Autodesk Inventor part; units mm, degrees
ref_plane "YZ Plane" through (0, 0, 0) normal (1, 0, 0) x (0, 1, 0)
ref_plane "XZ Plane" through (0, 0, 0) normal (0, 1, 0) x (-1, 0, 0)
ref_plane "XY Plane" through (0, 0, 0) normal (0, 0, 1) x (1, 0, 0)
sketch "Sketch1" plane through (0, 0, 0) normal (0, 1, 0) x (-1, 0, 0)
  line L0 (0, 0) -> (-32, 0)
  line L1 (-32, 0) -> (-32, -24)
  line L2 (-32, -24) -> (0, -24)
  line L3 (0, -24) -> (0, 0)
  circle A0 centre (-8.5, -19) radius 2
  circle A1 centre (-23.5, -19) radius 2
  circle A2 centre (-23.5, -5) radius 2
  circle A3 centre (-8.5, -5) radius 2
  line L4 (-16, -24) -> (-16, 0) construction
  line L5 (0, -12) -> (-32, -12) construction
  dimension "d0" = 32
  dimension "d1" = 24
  dimension "x" = 4
  dimension "d3" = 4
  dimension "d4" = 4
  dimension "d5" = 4
  dimension "d6" = 15
  dimension "d7" = 7.5
  dimension "d8" = 14
  dimension "d9" = 7
extrude "Extrusion1" add sketch "Sketch1" along normal blind 10
sketch "Sketch2" plane through (0, 10, 0) normal (0, 1, 0) x (1, 0, 0)
  circle A0 centre (23.5, 5) radius 2
  circle A1 centre (8.5, 19) radius 2
  circle A2 centre (23.5, 19) radius 2
  circle A3 centre (8.5, 5) radius 2
  circle A4 centre (8.5, 19) radius 3
  circle A5 centre (23.5, 19) radius 3
  circle A6 centre (8.5, 5) radius 3
  circle A7 centre (23.5, 5) radius 3
  point P0 (0, 0)
  dimension "d12" = 6
  dimension "d13" = 6
  dimension "d14" = 6
  dimension "d15" = 6
extrude "Extrusion2" cut sketch "Sketch2" against normal blind 2.5 contours A3 | A4 | A5 | A6 | A7
equation "\"d3\" = x"
equation "\"d4\" = x"
equation "\"d5\" = x"
properties part number "WristMotorTensioner"
Could you check a few things on this model? Use its own coordinates, in mm. A direction names the side the tool comes from. Round coordinates to 2 decimals unless told otherwise and drop trailing zeros. Write each loop counter-clockwise with the first axis right and the second up, starting at its lowest first coordinate (ties: lowest second). Pieces come first, ordered by that corner, then holes.
(1) Suppose I cut it at B-B on x = 23.5. Write out the boundary of the cut face in (y, z).
Findings below:
outline: (0, -24) - (10, -24) - (10, -22) - (7.5, -22) - (7.5, -21) - (0, -21) - close; (0, -17) - (7.5, -17) - (7.5, -16) - (10, -16) - (10, -8) - (7.5, -8) - (7.5, -7) - (0, -7) - close; (0, -3) - (7.5, -3) - (7.5, -2) - (10, -2) - (10, 0) - (0, 0) - close
(2) If I drill on probe 1 along Z at (x, y) = (8.5, 4); probe 2 along X at (y, z) = (9, -5); probe 3 along Z at (x, y) = (8.5, 8.3), over which ranges is the centre line in solid material (lowest first)?
Findings below:
probe 1: z = -24 to -21, -17 to -7, -3 to 0
probe 2: x = 0 to 5.5, 11.5 to 20.5, 26.5 to 32
probe 3: z = -24 to -22, -16 to -8, -2 to 0
(3) For pin 1 (5 mm diameter, centred on x = 23.5, z = -5, fed in from -Y); pin 2 (5 mm diameter, centred on x = 8.5, z = -5, fed in from +Y), each with a flat end and sliding along its axis, tell me the tip position at first contact or that it passes through.
Findings below:
pin 1: stops at y = 0
pin 2: stops at y = 7.5
(4) Thinking about a two-plate mould opening in Z: for faces 3 (the face through (16, 5, -24)), 4 (the face through (21, 7.5, -19)), 5 (the face through (16, 10, -12)), which applies, +Z half, -Z half, draft (parallel to the pull), parting line (faces both ways), or undercut?
Findings below:
face 3: -Z half
face 4: undercut
face 5: draft
(5) Which directions (+Z, -Z, +X, -X, +Y, -Y) give clear straight access to the entire face, cutting with the end or side of a thin tool? Please do faces 1 (the face through (0, 5, -12)), 2 (the face through (21.1, 8.8, -17.2)).
Findings below:
face 1: +Z, -Z, -X, +Y, -Y
face 2: +Y
(6) Suppose I cut it at D-D on y = 8. Write out the boundary of the cut face in (x, z).
Findings below:
outline: (0, -24) - (32, -24) - (32, 0) - (0, 0) - close; hole circle Ø6 at (8.5, -19); hole circle Ø6 at (8.5, -5); hole circle Ø6 at (23.5, -19); hole circle Ø6 at (23.5, -5)
(7) Suppose I cut it at C-C on y = 3.25. Write out the boundary of the cut face in (x, z), and give its area (3 significant figures).
Findings below:
outline: (0, -24) - (32, -24) - (32, 0) - (0, 0) - close; hole circle Ø4 at (8.5, -19); hole circle Ø4 at (8.5, -5); hole circle Ø4 at (23.5, -19); hole circle Ø4 at (23.5, -5)
area: 718 mm2
(8) Suppose I cut it at A-A on z = -5. Write out the boundary of the cut face in (x, y).
Findings below:
outline: (0, 0) - (6.5, 0) - (6.5, 7.5) - (5.5, 7.5) - (5.5, 10) - (0, 10) - close; (10.5, 0) - (21.5, 0) - (21.5, 7.5) - (20.5, 7.5) - (20.5, 10) - (11.5, 10) - (11.5, 7.5) - (10.5, 7.5) - close; (25.5, 0) - (32, 0) - (32, 10) - (26.5, 10) - (26.5, 7.5) - (25.5, 7.5) - close
